Part model, mm, in its own coordinate system. Face numbers are marked on the shaded views. Round coordinates to 2 decimals unless told otherwise and drop trailing zeros. Write each loop counter-clockwise with the first axis right and the second up, starting at its lowest first coordinate (ties: lowest second). Pieces come first, ordered by that corner, then holes. Notation, with made-up numbers: M 18.5,75 L 55.5,75 A32 cw 55.5,103 Z; hole C -14,84.25 d10. An arc over 180 degrees is marked long. Use a Markdown table: item, result. Add a question column.
1) Slice it at A-A on x = 0. Write the cut outline in (y, z), plus the area to 3 significant figures.
2) Slice it at B-B on z = 18. Write the cut outline in (x, y) (3 decimals), plus the area to 3 significant figures.
3) Slice it at C-C on y = 3.75. Write the cut outline in (x, z), plus the area to 3 significant figures.
4) Two-plate mould, pull along X, no slides. Class the marked faces 1 and 2: released by +X, released by -X, zero draft, split by the parting line, or undercut.
5) Drop flat-ended pins along their axis: P1, Ø2, axis at y = -1.5, z = 16.5, coming from the -X side; P2, Ø3, axis at y = -1, z = 16, coming from the +X side; P3, Ø1.7, axis at x = -0.5, y = 3, coming from the +Z side; P4, Ø1.5, axis at y = 2, z = 5, coming from the -X side. Give the stop position or say it passes through.
6) Wall check: probe 1 along Y at (x, z) = (0.75, 15.5); probe 2 along Y at (x, z) = (-2, 5.75); probe 3 along Z at (x, y) = (2.5, 1.5). Give the ranges that are in metal, low to high.
```python
from build123d import *

# Parameters (mm, degrees)
SKETCH2_R           = 4
BOSS_EXTRUDE1_DEPTH = 28
CUT_EXTRUDE1_DEPTH  = 20.5
CHAMFER2_SIZE       = 0.5


with BuildPart() as part:
    # Sketch2 → Boss-Extrude1 (new body)
    with BuildSketch(Plane.XY):
        Circle(SKETCH2_R)
    extrude(amount=BOSS_EXTRUDE1_DEPTH)

    # Sketch4 → Cut-Extrude1 (cut)
    with BuildSketch(Plane.XY.offset(28)):
        Polygon((-3.475, 1.981003534), (3.475, 1.981003534), (3.475, 4), (0, 4), (-3.475, 4), align=None)
    extrude(amount=-CUT_EXTRUDE1_DEPTH, mode=Mode.SUBTRACT)

    # Chamfer2
    chamfer2_edges = [part.edges().sort_by_distance(p)[0] for p in [
        (0, 1.981003534, 7.5),
        (-1.024695077, -3.866522986, 28),
        (0, 1.981003534, 28),
    ]]
    chamfer(chamfer2_edges, length=CHAMFER2_SIZE)


solid = part.part
```
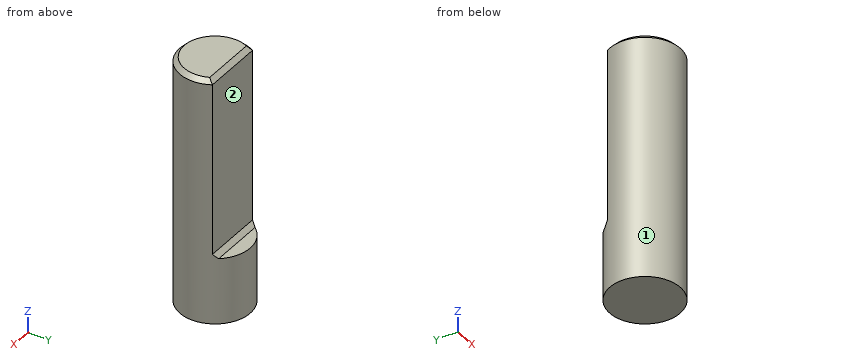
Entries:
| question | item | result |
|---|---|---|
| 1 | outline | M -4,0 L 4,0 L 4,7.5 L 2.48,7.5 L 1.98,8 L 1.98,27.5 L 1.48,28 L -3.5,28 L -4,27.5 Z |
| 1 | area | 182 mm^2 |
| 2 | outline | M -3.475,1.981 A4 ccw long 3.475,1.981 Z |
| 2 | area | 40.3 mm^2 |
| 3 | outline | M -1.39,0 L 1.39,0 L 1.39,7.5 L -1.39,7.5 Z |
| 3 | area | 20.9 mm^2 |
| 4 | face 1 | split by the parting line |
| 4 | face 2 | zero draft |
| 5 | P1 | stops at x = -3.97 |
| 5 | P2 | stops at x = 4 |
| 5 | P3 | stops at z = 7.83 |
| 5 | P4 | stops at x = -3.8 |
| 6 | probe 1 | y = -3.93 to 1.98 |
| 6 | probe 2 | y = -3.46 to 3.46 |
| 6 | probe 3 | z = 0 to 27.98 |
